Verification items for the finished model (mm, model axes). Face numbers are marked on the shaded views. A direction names the side the tool comes from. Coordinates: 2 decimals unless noted, no trailing zeros. Write each loop counter-clockwise with the first axis right and the second up, starting at its lowest first coordinate (ties: lowest second). Pieces come first, ordered by that corner, then holes. Notation, with made-up numbers: (82, 60.25) -> (87, 60.25) arc R10 ccw to (87, 68.25) -> close; hole circle Ø5 at (-2.75, -26.75). An arc over 180 degrees is marked (long way). Use CSV: the item, a comma, the result in double quotes.
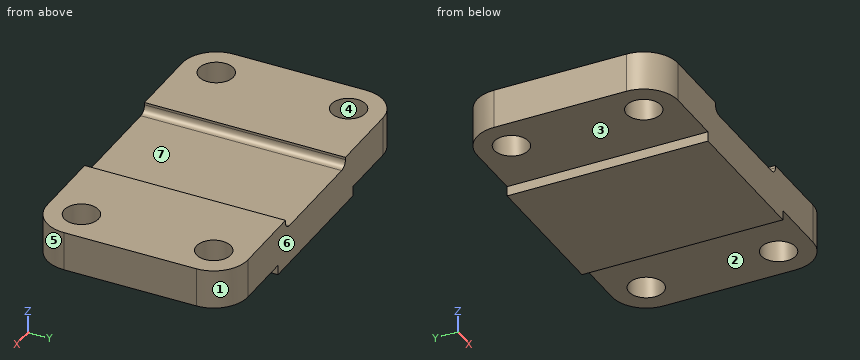
```python
from build123d import *

# Parameters (mm, degrees)
F1_DEPTH = 82
F2_R     = 3
F3_R     = 7
F4_DEPTH = 16.001
F5_R     = 14


with BuildPart() as f1:
    # F0 (on Front) → F1 (new body)
    with BuildSketch(Plane.XZ):
        Polygon((0, 16), (0, 0), (38, 0), (38, -4), (98, -4), (98, 0), (136, 0), (136, 16), (92, 16), (92, 12), (44, 12), (44, 16), align=None)
    extrude(amount=-F1_DEPTH)

    # F2
    f2_edges = [f1.edges().sort_by_distance(p)[0] for p in [
        (44, 41, 12),
        (92, 41, 12),
    ]]
    fillet(f2_edges, radius=F2_R)

    # F3 (on Top) → F4 (cut, through all)
    with BuildSketch(Plane.XY):
        with Locations((14, 14)):
            Circle(F3_R)
        with Locations((122, 14)):
            Circle(F3_R)
        with Locations((14, 68)):
            Circle(F3_R)
        with Locations((122, 68)):
            Circle(F3_R)
    extrude(amount=F4_DEPTH, mode=Mode.SUBTRACT)

    # F5
    f5_edges = [f1.edges().sort_by_distance(p)[0] for p in [
        (0, 0, 8),
        (0, 82, 8),
        (136, 0, 8),
        (136, 82, 8),
    ]]
    fillet(f5_edges, radius=F5_R)


solid = f1.part
```
1) Cross-section at D-D (x = 64). Record the boundary of the cut face in (y, z), plus the area to 3 significant figures.
Return value:
outline,"(0, -4) -> (82, -4) -> (82, 12) -> (0, 12) -> close"
area,"1,310 mm2"
2) Set-up check for the marked faces 1, 2 and 3: record each of +Z, -Z, +X, -X, +Y, -Y from which the full face is reachable in a straight line by a thin tool's end or side.
Return value:
face 1,"+Z, -Z, +X, +Y"
face 2,"-Z, +X, +Y, -Y"
face 3,"-Z, -X, +Y, -Y"
3) Cross-section at C-C (y = 33.5). Record the boundary of the cut face in (x, z), plus the area to 3 significant figures.
Return value:
outline,"(0, 0) -> (38, 0) -> (38, -4) -> (98, -4) -> (98, 0) -> (136, 0) -> (136, 16) -> (92, 16) -> (92, 15) arc R3 cw to (89, 12) -> (47, 12) arc R3 cw to (44, 15) -> (44, 16) -> (0, 16) -> close"
area,"2,230 mm2"
4) Cross-section at A-A (z = 2.25). Record the boundary of the cut face in (x, y).
Return value:
outline,"(0, 14) arc R14 ccw to (14, 0) -> (122, 0) arc R14 ccw to (136, 14) -> (136, 68) arc R14 ccw to (122, 82) -> (14, 82) arc R14 ccw to (0, 68) -> close; hole circle Ø14 at (14, 14); hole circle Ø14 at (14, 68); hole circle Ø14 at (122, 14); hole circle Ø14 at (122, 68)"
5) Mould release check, pull along X, two halves, no side actions. Record for the marked faces 4, 5, 6 and 7: released by +X, released by -X, zero draft, split by the parting line, or undercut.
Return value:
face 4,"undercut"
face 5,"released by +X"
face 6,"zero draft"
face 7,"undercut"
6) Gauge pin test, flat ends, axial feed: pin 1 (16 mm diameter, centred on x = 122, y = 14, fed in from -Z); pin 2 (12 mm diameter, centred on x = 94, z = 6, fed in from -Y); pin 3 (4 mm diameter, centred on x = 83, y = 50.5, fed in from +Z); pin 4 (1.2 mm diameter, centred on y = 36, z = -1.5, fed in from +X). Record the tip position at first contact, or that the pin passes through.
Return value:
pin 1,"z = 0"
pin 2,"y = 0"
pin 3,"z = 12"
pin 4,"x = 98"
7) Scan lines: L1, parallel to Y at x = 14, z = 5.5; L2, parallel to X at y = 14, z = 3; L3, parallel to X at y = 9, z = 1.75. Record each from-to range of solid material in increasing order.
Return value:
L1,"0 to 7, 21 to 61, 75 to 82"
L2,"0 to 7, 21 to 115, 129 to 136"
L3,"0.92 to 9.1, 18.9 to 117.1, 126.9 to 135.08"
8) Cross-section at B-B (y = 18.5). Record the boundary of the cut face in (x, z).
Return value:
outline,"(0, 0) -> (8.64, 0) -> (8.64, 16) -> (0, 16) -> close; (19.36, 0) -> (38, 0) -> (38, -4) -> (98, -4) -> (98, 0) -> (116.64, 0) -> (116.64, 16) -> (92, 16) -> (92, 15) arc R3 cw to (89, 12) -> (47, 12) arc R3 cw to (44, 15) -> (44, 16) -> (19.36, 16) -> close; (127.36, 0) -> (136, 0) -> (136, 16) -> (127.36, 16) -> close"
